The listing builds one solid part. Answer for the finished solid, in the listing's coordinates (mm). A direction names the side the tool comes from. Coordinates: 2 decimals unless noted, no trailing zeros. Order: outer loops, then holes, each group sorted by start corner. A loop starts at its lowest first (then second) coordinate and runs counter-clockwise, first axis right, second up. Notation, with made-up numbers: (69.25, -27.75) - (118.25, -27.75) arc R29 ccw to (118.25, -2.75) - close; hole circle Ø6 at (26.25, 51). An arc over 180 degrees is marked (long way). Use a Markdown table: item, result. Add a question column.
Item 1: Find the intervals of material crossed by line 1 along X through (y, z) = (-2, 21); line 2 along Y through (x, z) = (1.25, 24.5); line 3 along Z through (x, y) = (0.75, 7), in increasing order.
Item 2: The part is cut by section D-D, the plane z = 6.6. State how many separate pieces and enclosed holes the cut face has, then the cut area to 3 significant figures.
Item 3: The mould has two halves that part along Y. Classify faces 1 (the flat face through (3.465, 12.493, -11.461)), 2 (the flat face through (7, 10, -1)), 3 (the flat face through (3, -5, 13)), 4 (the flat face through (2.4, 0, 4.6)): released by +Y, released by -Y, zero draft, split by the parting line, or undercut.
Item 4: The part is cut by section B-B, the plane x = 3.5. Give the vertices of the cut face in (y, z), then the cut area to 3 significant figures.
Item 5: The part is cut by section A-A, the plane z = 21.6. Give the vertices of the cut face in (x, y).
Item 6: Flat-ended cylindrical pins translate along their axes: P1, Ø3.5, axis at x = 3.5, z = 6.6, coming from the -Y side; P2, Ø2.5, axis at x = 4.5, z = 7.5, coming from the +Y side; P3, Ø2, axis at y = 19, z = -5.5, coming from the -X side; P4, Ø1.5, axis at x = 5.5, z = -27, coming from the -Y side. Find the tip coordinate at first contact, or state that the pin passes through.
Item 7: The part is cut by section C-C, the plane y = -3. Give the vertices of the cut face in (x, z).
Item 8: For faces 5 (the flat face through (3, -3, 0)), 6 (the cylindrical face through (6.699, 12.444, -10.609)), 7 (the flat face through (3, 2, 11.1)), determine the directions among +Z, -Z, +X, -X, +Y, -Y from which every point of the face is accessible in a straight line to the end or side of a thin tool.
from build123d import *

# Parameters (mm, degrees)
BOSS_EXTRUDE1_DEPTH = 7
FILLET1_R           = 1
SKETCH2_R           = 2.1
CUT_EXTRUDE1_DEPTH  = 7


with BuildPart() as part:
    # Sketch1 → Boss-Extrude1 (new body)
    with BuildSketch(Plane.YZ):
        Polygon((0, 0), (-5, 0), (-5, 28.2), (0, 28.2), (0, 17.1), (6.992997501, 17.1), (27.73775651, -32.237200317), (28.226677629, -33.4), (21.717869147, -33.4), (3.007002499, 11.1), (0, 11.1), align=None)
    extrude(amount=BOSS_EXTRUDE1_DEPTH)

    # Fillet1
    fillet1_edges = [part.edges().sort_by_distance(p)[0] for p in [
        (0, 0, 5.55),
        (0, -2.5, 0),
        (0, -2.5, 28.2),
        (0, 0, 22.65),
        (0, 3.49649875, 17.1),
        (0, 17.609837565, -8.15),
        (0, 12.362435823, -11.15),
        (0, 1.50350125, 11.1),
        (7, 17.609837565, -8.15),
        (3.5, 0, 11.1),
        (3.5, 0, 0),
        (3.5, -5, 28.2),
        (3.5, 0, 28.2),
        (3.5, 0, 17.1),
        (3.5, 6.992997501, 17.1),
        (7, 3.49649875, 17.1),
        (7, 0, 22.65),
        (7, -2.5, 28.2),
        (7, -2.5, 0),
        (7, 0, 5.55),
        (7, 1.50350125, 11.1),
        (7, 12.362435823, -11.15),
    ]]
    fillet(fillet1_edges, radius=FILLET1_R)

    # Sketch2 → Cut-Extrude1 (cut)
    with BuildSketch(Plane.XZ.offset(5)):
        with Locations(Location((3.5, 21.6, 0), (0, 0, 270))):
            Circle(SKETCH2_R)
        with Locations(Location((3.5, 6.6, 0), (0, 0, 270))):
            Circle(SKETCH2_R)
    extrude(amount=-CUT_EXTRUDE1_DEPTH, mode=Mode.SUBTRACT)


solid = part.part
Solution:
| question | item | result |
|---|---|---|
| 1 | line 1 | x = 0 to 1.49, 5.51 to 7 |
| 1 | line 2 | y = -5 to 0 |
| 1 | line 3 | z = 1.69 to 16.8 |
| 2 | separate pieces | 3 |
| 2 | enclosed holes | 0 |
| 2 | area | 58.2 mm2 |
| 3 | face 1 | undercut |
| 3 | face 2 | zero draft |
| 3 | face 3 | released by -Y |
| 3 | face 4 | undercut |
| 4 | outline | (-5, 0) - (-1, 0) arc R1 ccw to (0, 1) - (0, 4.5) - (-5, 4.5) - close; (-5, 8.7) - (0, 8.7) - (0, 10.1) arc R1 cw to (1, 11.1) - (3.01, 11.1) - (21.72, -33.4) - (28.23, -33.4) - (7.25, 16.49) arc R1 ccw to (6.33, 17.1) - (1, 17.1) arc R1 cw to (0, 18.1) - (0, 19.5) - (-5, 19.5) - close; (-5, 23.7) - (0, 23.7) - (0, 27.2) arc R1 ccw to (-1, 28.2) - (-4, 28.2) arc R1 ccw to (-5, 27.2) - close |
| 4 | area | 438 mm2 |
| 5 | outline | (0, -5) - (1.4, -5) - (1.4, 0) - (1, 0) arc R1 ccw to (0, -1) - close; (5.6, -5) - (7, -5) - (7, -1) arc R1 ccw to (6, 0) - (5.6, 0) - close |
| 6 | P1 | stops at y = 4.16 |
| 6 | P2 | stops at y = 11.56 |
| 6 | P3 | passes through |
| 6 | P4 | stops at y = 18.71 |
| 7 | outline | (0, 1) arc R1 ccw to (1, 0) - (6, 0) arc R1 ccw to (7, 1) - (7, 27.2) arc R1 ccw to (6, 28.2) - (1, 28.2) arc R1 ccw to (0, 27.2) - close; hole circle Ø4.2 at (3.5, 6.6); hole circle Ø4.2 at (3.5, 21.6) |
| 8 | face 5 | -Z, +X, -X, -Y |
| 8 | face 6 | -Z, +X |
| 8 | face 7 | -Z, +X, -X |
